Design review of the part built by this model. Coordinates are the model's own, in mm. Face numbers are marked on the shaded views. A direction names the side the tool comes from. Coordinates: 2 decimals unless noted, no trailing zeros. Loops run counter-clockwise (first coordinate to the right, second up) from the corner with the lowest first, then second, coordinate; pieces in that order, holes last.
Q1. Add section C-C on y = 424. Give the boundary of the cut face in (x, z).
Q2. Add section B-B on z = -1039. Give the boundary of the cut face in (x, y), and give its area (3 significant figures).
Q3. Add section A-A on x = 794. Give the boundary of the cut face in (y, z), and give its area (3 significant figures).
Q4. For P1, Ø1.5, axis at x = 342, z = -175, coming from the -Y side; P2, Ø8, axis at x = 1513, y = 733, coming from the +Z side (3 decimals); P3, Ø10, axis at x = 868.5, z = -395.5, coming from the +Y side; P4, Ø6, axis at x = 539, z = -186.5, coming from the +Y side, all flat-tipped, find the tip position at first contact; note any pin that passes through.
Q5. Machinability: for the marked faces 1, 2 and 3, which of the approach directions +Z, -Z, +X, -X, +Y, -Y give a long, thin tool a straight path to every point of the face, cutting with its end or side? Answer none if there is none.
Q6. Add section D-D on x = 1204. Give the boundary of the cut face in (y, z), and give its area (3 significant figures).
Q7. Wall thickness on probe 1 along X at (y, z) = (1173.5, -568); probe 2 along X at (y, z) = (1186.5, -967); probe 3 along Z at (x, y) = (859.5, 733) (3 decimals): over which ranges is each line inside the solid? List them lowest first.
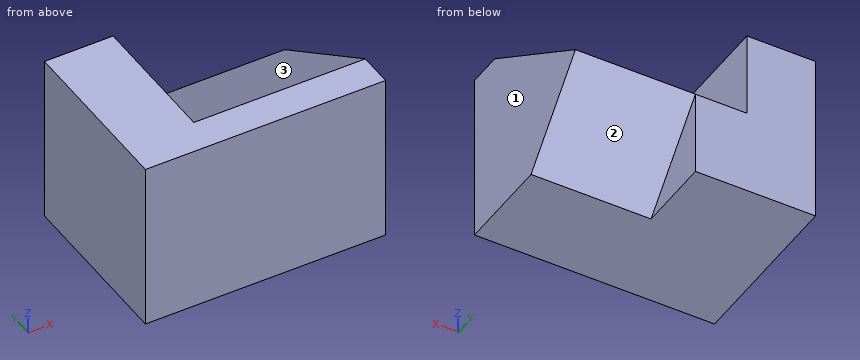
```python
from build123d import *

# Parameters (mm, degrees)
SKETCH1_W               = 1778
SKETCH1_H               = 1270
BOSS_EXTRUDE1_DEPTH     = 1270
CUT_EXTRUDE1_DEPTH      = 2528.268090251
CUT_EXTRUDE1_DEPTH_BACK = 1270
CUT_EXTRUDE2_DEPTH      = 2528.268090251
CUT_EXTRUDE2_DEPTH_BACK = 889


with BuildPart() as part:
    # Sketch1 → Boss-Extrude1 (new body)
    with BuildSketch(Plane(origin=(0, 0, 0), x_dir=(1, 0, 0), z_dir=(0, 1, 0))):
        with Locations((889, 635)):
            Rectangle(SKETCH1_W, SKETCH1_H)
    extrude(amount=BOSS_EXTRUDE1_DEPTH)

    # Sketch2 → Cut-Extrude1 (cut, two sides: drawn at the far end of the back side and taken through both)
    with BuildSketch(Plane(origin=(1778, 0, 0), x_dir=(0, 0, -1), z_dir=(1, 0, 0)).offset(-CUT_EXTRUDE1_DEPTH_BACK)):
        Polygon((0, 254), (635, 1270), (0, 1270), align=None)
    extrude(amount=CUT_EXTRUDE1_DEPTH + CUT_EXTRUDE1_DEPTH_BACK, mode=Mode.SUBTRACT)

    # Sketch2<4> → Cut-Extrude2 (cut, two sides: drawn at the far end of the back side and taken through both)
    with BuildSketch(Plane(origin=(1778, 0, 0), x_dir=(0, 0, -1), z_dir=(1, 0, 0)).offset(-CUT_EXTRUDE2_DEPTH_BACK)):
        Polygon((1270, 1270), (635, 1270), (1270, 711.2), align=None)
    extrude(amount=CUT_EXTRUDE2_DEPTH + CUT_EXTRUDE2_DEPTH_BACK, mode=Mode.SUBTRACT)


solid = part.part
```
Entries:
1. outline: (0, -1270) - (1778, -1270) - (1778, -106.25) - (508, -106.25) - (508, 0) - (0, 0) - close
2. outline: (0, 0) - (1778, 0) - (1778, 914.48) - (889, 914.48) - (889, 1270) - (0, 1270) - close
2. area: 1,940,000 mm2
3. outline: (0, -1270) - (1270, -1270) - (1270, -635) - (254, 0) - (0, 0) - close
3. area: 1,290,000 mm2
4. P1: stops at y = 0
4. P2: stops at z = -296.875
4. P3: stops at y = 894.8
4. P4: stops at y = 557.2
5. face 1: +Z, -Z, +X, +Y, -Y
5. face 2: -Z, +X, +Y
5. face 3: +Z, +X, +Y
6. outline: (0, -1270) - (711.2, -1270) - (1270, -635) - (254, 0) - (0, 0) - close
6. area: 1,110,000 mm2
7. probe 1: x = 0 to 508
7. probe 2: x = 0 to 889
7. probe 3: z = -1270 to -299.375
